```python
from build123d import *


with BuildPart() as part:
    # Esquisse1 → Révol.-Mince2 (revolve)
    with BuildSketch(Plane.XY, mode=Mode.PRIVATE) as r_vol_mince2_sk:
        Polygon((2.76, 10.056278032), (2.76, 8.5), (0, 8.5), (0, 12.5), (3.26, 16), (3.991750138, 15.318427014), (1, 12.106425332), (1, 9.5), (1.76, 9.5), (1.76, 10.056278032), align=None)
    revolve(r_vol_mince2_sk.sketch.rotate(Axis((-7.892655367, 0, 0), (1, 0, 0)), 90), axis=Axis((-7.892655367, 0, 0), (1, 0, 0)))


solid = part.part
```
Source: CAD feature listing. Evaluate the final solid. Frame: model axes, mm. A direction names the side the tool comes from. Round coordinates to 2 decimals unless told otherwise and drop trailing zeros. Loops run counter-clockwise (first coordinate to the right, second up) from the corner with the lowest first, then second, coordinate; pieces in that order, holes last. Notation, with made-up numbers: M -1,45 L 44,45 A16 ccw 44,57 Z; hole C 29,2 d3. An arc over 180 degrees is marked long. Use a Markdown table: item, result. Add a question column.
1. Contact query for flat-ended pins moving along their axis: P1, Ø12, axis at y = 7.5, z = -4, coming from the +X side; P2, Ø1.5, axis at y = 6.5, z = -12.5, coming from the -X side; P3, Ø10, axis at y = 5, z = 3.5, coming from the +X side; P4, Ø16, axis at y = 4.5, z = -0.5, coming from the -X side. Output: stop coordinate, or through.
2. Reachability of faces 4 (the cylindrical face through (2.267, 9.817, -2.18)), 5 (the flat face through (1, 5.3, -8.1)) from +Z, -Z, +X, -X, +Y, -Y: full face, straight path, thin tool, end or side. Return the list, or none.
3. Line query: line 1 (Z direction, x = 1.7, y = -5); line 2 (Y direction, x = 2.25, z = -7); line 3 (Y direction, x = 1.85, z = 7.5). Output: solid intervals per line, ascending.
4. Section query A-A on z = 0. Return the cut outline in (x, y).
5. Mould query, pull axis Z, two halves, no side actions, for faces 1 (the flat face through (0, 8.2, 3)), 2 (the conical face through (0.2, 12.4, -2.8)), 3 (the cylindrical face through (1.361, -8.428, -1.107)). Classes: pulls with the +Z half, pulls with the -Z half, needs draft (parallel to the pull), parting line crosses it, or undercut.
Reported:
| question | item | result |
|---|---|---|
| 1 | P1 | stops at x = 3.23 |
| 1 | P2 | stops at x = 0.78 |
| 1 | P3 | stops at x = 2.76 |
| 1 | P4 | stops at x = 0 |
| 2 | face 4 | +X |
| 2 | face 5 | none |
| 3 | line 1 | z = -13.42 to -11.85, -8.08 to -6.87, 6.87 to 8.08, 11.85 to 13.42 |
| 3 | line 2 | y = -13.17 to -11.48, -7.22 to -4.82, 4.82 to 7.22, 11.48 to 13.17 |
| 3 | line 3 | y = -12.39 to -10.64, -6.7 to -4, 4 to 6.7, 10.64 to 12.39 |
| 4 | outline | M 0,-12.5 L 3.26,-16 L 3.99,-15.32 L 1,-12.11 L 1,-9.5 L 1.76,-9.5 L 1.76,-10.06 L 2.76,-10.06 L 2.76,-8.5 L 0,-8.5 Z; M 0,8.5 L 2.76,8.5 L 2.76,10.06 L 1.76,10.06 L 1.76,9.5 L 1,9.5 L 1,12.11 L 3.99,15.32 L 3.26,16 L 0,12.5 Z |
| 5 | face 1 | needs draft |
| 5 | face 2 | parting line crosses it |
| 5 | face 3 | undercut |
